Can you work these out from the model? Positions are in its coordinate system, mm. Face numbers are marked on the shaded views. Give positions to 0.01 mm unless a question says otherwise; leave off trailing zeros. Order: outer loops, then holes, each group sorted by start corner. A loop starts at its lowest first (then second) coordinate and runs counter-clockwise, first axis right, second up. Notation, with made-up numbers: (-28.75, 49.5) - (-20.75, 49.5) arc R9 cw to (-20.75, 60.5) - close; hole circle Ø5 at (56, 38). An arc over 180 degrees is marked (long way). Use one line per item in the form item = value. Start each with the question number.
1) Please list where these lines run through material, in increasing order: probe 1 along Z at (x, y) = (7, -6); probe 2 along X at (y, z) = (-6.5, 11); probe 3 along Z at (x, y) = (7.5, -13.75).
2) For pin 1 (1.5 mm diameter, centred on x = -3.5, z = 10, fed in from -Y), with a flat end and sliding along its axis, tell me the tip position at first contact or that it passes through.
3) Suppose I cut it at D-D, the plane x = 6.5. Write out the boundary of the cut face in (y, z), and give its area (3 significant figures).
4) We'd pull the mould along X, two halves only. Please class the marked faces 1, 2 and 3: released by +X, released by -X, zero draft, split by the parting line, or undercut.
5) Suppose I cut it at C-C, the plane x = -1. Write out the boundary of the cut face in (y, z).
6) Suppose I cut it at B-B, the plane z = 11. Write out the boundary of the cut face in (x, y).
7) Suppose I cut it at A-A, the plane y = -4. Write out the boundary of the cut face in (x, z).
```python
from build123d import *

# Parameters (mm, degrees)
SKETCH_1_R          = 1.5
EXTRUDE_1_DEPTH     = 14
SKETCH_2_R          = 1.25
CUT_EXTRUDE_1_DEPTH = 15


with BuildPart() as part:
    # 草图1 → 凸台-拉伸1 (new body)
    with BuildSketch(Plane.XY):
        Polygon((-5, -10), (0, -15), (10, -15), (10, 0), (-5, 0), align=None)
        with Locations((-1, -4)):
            Circle(SKETCH_1_R, mode=Mode.SUBTRACT)
    extrude(amount=EXTRUDE_1_DEPTH)

    # 草图2 → 切除-拉伸1 (cut)
    with BuildSketch(Plane(origin=(0, 0, 0), x_dir=(1, 0, 0), z_dir=(0, 1, 0))):
        with Locations(Location((6.5, -3, 0), (0, 0, 270))):
            Circle(SKETCH_2_R)
        with Locations(Location((6.5, -11, 0), (0, 0, 270))):
            Circle(SKETCH_2_R)
    extrude(amount=-CUT_EXTRUDE_1_DEPTH, mode=Mode.SUBTRACT)


solid = part.part
```
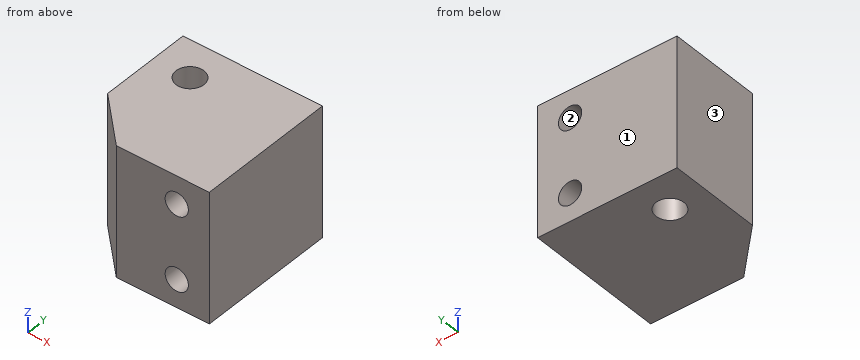
Result sheet:
q1.probe_1 = 0 to 1.85, 4.15 to 9.85, 12.15 to 14
q1.probe_2 = -5 to 5.25, 7.75 to 10
q1.probe_3 = 0 to 2.25, 3.75 to 10.25, 11.75 to 14
q2.pin_1 = -12.25
q3.outline = (-15, 0) - (0, 0) - (0, 1.75) - (-15, 1.75) - close; (-15, 4.25) - (0, 4.25) - (0, 9.75) - (-15, 9.75) - close; (-15, 12.25) - (0, 12.25) - (0, 14) - (-15, 14) - close
q3.area = 135 mm²
q4.face_1 = zero draft
q4.face_2 = undercut
q4.face_3 = released by -X
q5.outline = (-14, 0) - (-5.5, 0) - (-5.5, 14) - (-14, 14) - close; (-2.5, 0) - (0, 0) - (0, 14) - (-2.5, 14) - close
q6.outline = (-5, -10) - (0, -15) - (5.25, -15) - (5.25, 0) - (-5, 0) - close; (7.75, -15) - (10, -15) - (10, 0) - (7.75, 0) - close; hole circle Ø3 at (-1, -4)
q7.outline = (-5, 0) - (-2.5, 0) - (-2.5, 14) - (-5, 14) - close; (0.5, 0) - (10, 0) - (10, 14) - (0.5, 14) - close; hole circle Ø2.5 at (6.5, 3); hole circle Ø2.5 at (6.5, 11)
